```python
from build123d import *

# Parameters (mm, degrees)
F0_W          = 124.7
F0_H          = 107
F0_W_2        = 122
F0_H_2        = 102
F0_W_3        = 1.3
F1_DEPTH      = 2
F2_DEPTH      = 7.2
F3_DEPTH      = 1
F3_DEPTH_BACK = 2


with BuildPart() as f1:
    # F0 (on Front) → F1 (new body)
    with BuildSketch(Plane.XZ):
        Polygon((-77.1, -57.5), (61.7, -57.5), (61.7, -55.5), (-65, -55.5), (-65, 55.5), (61.7, 55.5), (61.7, 57.5), (-77.1, 57.5), align=None)
        Polygon((61.7, -53.5), (61.7, -55.5), (65, -55.5), (65, 55.5), (61.7, 55.5), (61.7, 53.5), (63, 53.5), (63, -53.5), align=None)
        Polygon((-65, -55.5), (61.7, -55.5), (61.7, -53.5), (-63, -53.5), (-63, 53.5), (61.7, 53.5), (61.7, 55.5), (-65, 55.5), align=None)
        with Locations((-0.65, 0)):
            Rectangle(F0_W, F0_H)
        with Locations((-0.3, 0)):
            Rectangle(F0_W_2, F0_H_2, mode=Mode.SUBTRACT)
        Polygon((61.7, -57.5), (66.5, -57.5), (66.5, 57.5), (61.7, 57.5), (61.7, 55.5), (65, 55.5), (65, -55.5), (61.7, -55.5), align=None)
        with Locations((62.35, 0)):
            Rectangle(F0_W_3, F0_H)
    extrude(amount=-F1_DEPTH)

    # F0 (on Front) → F2 (join)
    with BuildSketch(Plane.XZ):
        Polygon((61.7, -53.5), (61.7, -55.5), (65, -55.5), (65, 55.5), (61.7, 55.5), (61.7, 53.5), (63, 53.5), (63, -53.5), align=None)
        Polygon((-65, -55.5), (61.7, -55.5), (61.7, -53.5), (-63, -53.5), (-63, 53.5), (61.7, 53.5), (61.7, 55.5), (-65, 55.5), align=None)
    extrude(amount=-F2_DEPTH)

    # F0 (on Front) → F3 (cut, two sides)
    with BuildSketch(Plane.XZ) as f3_sk:
        Polygon((61.7, -57.5), (66.5, -57.5), (66.5, 57.5), (61.7, 57.5), (61.7, 55.5), (65, 55.5), (65, -55.5), (61.7, -55.5), align=None)
        with Locations((62.35, 0)):
            Rectangle(F0_W_3, F0_H)
        Polygon((61.7, -53.5), (61.7, -55.5), (65, -55.5), (65, 55.5), (61.7, 55.5), (61.7, 53.5), (63, 53.5), (63, -53.5), align=None)
    extrude(amount=-F3_DEPTH, mode=Mode.SUBTRACT)
    extrude(f3_sk.sketch, amount=F3_DEPTH_BACK, mode=Mode.SUBTRACT)


solid = f1.part
```
Geometry: final body of the model. Coordinates: model frame, mm. A direction names the side the tool comes from. Coordinates: 2 decimals unless noted, no trailing zeros. Order: outer loops, then holes, each group sorted by start corner. A loop starts at its lowest first (then second) coordinate and runs counter-clockwise, first axis right, second up. Notation, with made-up numbers: (-29.5, 84.5) -> (-1.5, 84.5) arc R15 cw to (-1.5, 102.5) -> close; hole circle Ø2 at (50, 53.5). An arc over 180 degrees is marked (long way). Write item = value, one per line.
(1) Pull-direction query (Z, two-part tool) for faces 4 (the flat face through (1, 5, -53.5)), 5 (the flat face through (0, 2, 52)), 6 (the flat face through (0, 7.2, 54)), 7 (the flat face through (1, 5, 55.5)); classes: pulls with the +Z half, pulls with the -Z half, needs draft (parallel to the pull), parting line crosses it, or undercut.
Solved:
face_4 = undercut
face_5 = undercut
face_6 = needs draft
face_7 = pulls with the +Z half
(2) Cut plane C-C on x = -15. Return loops of the section in (y, z), plus the area to 3 significant figures.
Solved:
outline = (0, -57.5) -> (2, -57.5) -> (2, -55.5) -> (7.2, -55.5) -> (7.2, -53.5) -> (2, -53.5) -> (2, -51) -> (0, -51) -> close; (0, 51) -> (2, 51) -> (2, 53.5) -> (7.2, 53.5) -> (7.2, 55.5) -> (2, 55.5) -> (2, 57.5) -> (0, 57.5) -> close
area = 46.8 mm²
(3) Cut plane A-A on z = -48. Return loops of the section in (x, y), plus the area to 3 significant figures.
Solved:
outline = (-77.1, 0) -> (-61.3, 0) -> (-61.3, 2) -> (-63, 2) -> (-63, 7.2) -> (-65, 7.2) -> (-65, 2) -> (-77.1, 2) -> close; (60.7, 0) -> (61.7, 0) -> (61.7, 1) -> (66.5, 1) -> (66.5, 2) -> (65, 2) -> (65, 7.2) -> (63, 7.2) -> (63, 2) -> (60.7, 2) -> close
area = 59.2 mm²
(4) Cut plane B-B on y = 3.75. Return loops of the section in (x, z).
Solved:
outline = (-65, -55.5) -> (65, -55.5) -> (65, 55.5) -> (-65, 55.5) -> close; hole (-63, -53.5) -> (63, -53.5) -> (63, 53.5) -> (-63, 53.5) -> close
(5) Cut plane D-D on x = -67. Return loops of the section in (y, z).
Solved:
outline = (0, -57.5) -> (2, -57.5) -> (2, 57.5) -> (0, 57.5) -> close
(6) Pin query (flat end, axial travel): pin 1 Ø4 at (x, y) = (27.5, 4.5) entering from +Z; pin 2 Ø1.5 at (y, z) = (5.5, -41.5) entering from +X; pin 3 Ø1.6 at (y, z) = (4, -3) entering from -X. Return the tip coordinate at first contact, or that it passes through.
Solved:
pin_1 = 55.5
pin_2 = 65
pin_3 = -65
(7) Access query for faces 1 (the flat face through (-65, 5, 1)), 2 (the flat face through (64, 1, 1)), 3 (the flat face through (63, 5, 1)). Directions: +Z, -Z, +X, -X, +Y, -Y. A direction counts if a zero-diameter tool reaches every point of the face in a straight line with its end or side. Return the directions, or none.
Solved:
face_1 = +Z, -Z, -X, +Y
face_2 = +Z, -Z, +X, -Y
face_3 = +Y
(8) Line query: line 1 (X direction, y = 2.5, z = -52); line 2 (Z direction, x = 59, y = 1); line 3 (X direction, y = 0.75, z = 41.5). Output: solid intervals per line, ascending.
Solved:
line_1 = -65 to -63, 63 to 65
line_2 = -57.5 to -51, 51 to 57.5
line_3 = -77.1 to -61.3, 60.7 to 61.7
